from build123d import *

# Parameters (mm, degrees)
SKETCH_1_R      = 37.5
SKETCH_1_R_2    = 2.05
SKETCH_1_R_3    = 5.05
SKETCH_1_W      = 8.1
SKETCH_1_H      = 2.1
EXTRUDE_1_DEPTH = 2


with BuildPart() as part:
    # 草图1 → 凸台-拉伸1 (new body)
    with BuildSketch(Plane.XY):
        with Locations((0, 26)):
            Circle(SKETCH_1_R)
        Circle(SKETCH_1_R_2, mode=Mode.SUBTRACT)
        with Locations((0, 8)):
            Circle(SKETCH_1_R_2, mode=Mode.SUBTRACT)
        with Locations((0, 26)):
            Circle(SKETCH_1_R_3, mode=Mode.SUBTRACT)
        with Locations((0, -7.5)):
            Circle(SKETCH_1_R_2, mode=Mode.SUBTRACT)
        with Locations((-15, 8)):
            Rectangle(SKETCH_1_W, SKETCH_1_H, mode=Mode.SUBTRACT)
        with Locations((-15, 0)):
            Rectangle(SKETCH_1_W, SKETCH_1_H, mode=Mode.SUBTRACT)
        with Locations((15, 8)):
            Rectangle(SKETCH_1_W, SKETCH_1_H, mode=Mode.SUBTRACT)
        with Locations((15, 0)):
            Rectangle(SKETCH_1_W, SKETCH_1_H, mode=Mode.SUBTRACT)
    extrude(amount=EXTRUDE_1_DEPTH)


solid = part.part
Check sheet for the modelled part. Datum: model origin and axes. Units: mm. Give positions to 0.01 mm unless a question says otherwise; leave off trailing zeros. Order: outer loops, then holes, each group sorted by start corner. A loop starts at its lowest first (then second) coordinate and runs counter-clockwise, first axis right, second up. Notation, with made-up numbers: M 5.25,83 L 61.25,83 A17 cw 61.25,101 Z; hole C -38,-37 d5. An arc over 180 degrees is marked long. Answer as CSV lines item,"result". Start each with the question number.
Item 1: Cross-section at A-A on y = 26. Enter the section's corners in (x, z), plus the area to 3 significant figures.
Item 2: Cross-section at B-B on x = 0. Enter the section's corners in (y, z).
Item 3: Mould release check, pull along X, two halves, no side actions. Record for faces 1 (the face through (10.95, 0, 1)), 2 (the face through (-8.13, -10.61, 0.99)), 3 (the face through (8, 27, 2)): +X half, -X half, draft (parallel to the pull), parting line (faces both ways), or undercut.
Item 4: Gauge pin test, flat ends, axial feed: P1, Ø0.6, axis at y = 0, z = 1, coming from the -X side; P2, Ø1, axis at x = -14, z = 1.5, coming from the -Y side; P3, Ø1, axis at x = 13.5, z = 0.5, coming from the -Y side; P4, Ø3.5, axis at x = 0, y = 0, coming from the -Z side. Record the tip position at first contact, or that the pin passes through.
Item 5: Cross-section at C-C on z = 1.6. State how many separate pieces and enclosed holes the cut face has, plus the area to 3 significant figures.
Item 6: Cross-section at D-D on x = 14.5. Enter the section's corners in (y, z), plus the area to 3 significant figures.
Item 7: Thickness scan on line 1 (Y direction, x = 0, z = 0.75); line 2 (Y direction, x = -16, z = 1.8); line 3 (Y direction, x = -18, z = 0.55). Record the ranges inside material, lowest first. Write a range as [from, to].
Established:
1,outline,"M -37.5,0 L -5.05,0 L -5.05,2 L -37.5,2 Z; M 5.05,0 L 37.5,0 L 37.5,2 L 5.05,2 Z"
1,area,"130 mm^2"
2,outline,"M -11.5,0 L -9.55,0 L -9.55,2 L -11.5,2 Z; M -5.45,0 L -2.05,0 L -2.05,2 L -5.45,2 Z; M 2.05,0 L 5.95,0 L 5.95,2 L 2.05,2 Z; M 10.05,0 L 20.95,0 L 20.95,2 L 10.05,2 Z; M 31.05,0 L 63.5,0 L 63.5,2 L 31.05,2 Z"
3,face 1,"undercut"
3,face 2,"parting line"
3,face 3,"draft"
4,P1,"stops at x = -27.31"
4,P2,"stops at y = -8.99"
4,P3,"stops at y = -9.17"
4,P4,"passes through"
5,separate pieces,"1"
5,enclosed holes,"8"
5,area,"4,230 mm^2"
6,outline,"M -8.58,0 L -1.05,0 L -1.05,2 L -8.58,2 Z; M 1.05,0 L 6.95,0 L 6.95,2 L 1.05,2 Z; M 9.05,0 L 60.58,0 L 60.58,2 L 9.05,2 Z"
6,area,"130 mm^2"
7,line 1,"y = [-11.5, -9.55], [-5.45, -2.05], [2.05, 5.95], [10.05, 20.95], [31.05, 63.5]"
7,line 2,"y = [-7.92, -1.05], [1.05, 6.95], [9.05, 59.92]"
7,line 3,"y = [-6.9, -1.05], [1.05, 6.95], [9.05, 58.9]"
